Check sheet for the drawn part. Datum: minimum x, y, z corner. Units: mm. Coordinates: 2 decimals unless noted, no trailing zeros. Order: outer loops, then holes, each group sorted by start corner. A loop starts at its lowest first (then second) coordinate and runs counter-clockwise, first axis right, second up. Notation, with made-up numbers: M 15.25,61 L 37.25,61 A5 cw 37.25,67 Z; hole C -13,-22.75 d5. An arc over 180 degrees is marked long. Use one line per item in the form item = value. Start each with the question number.
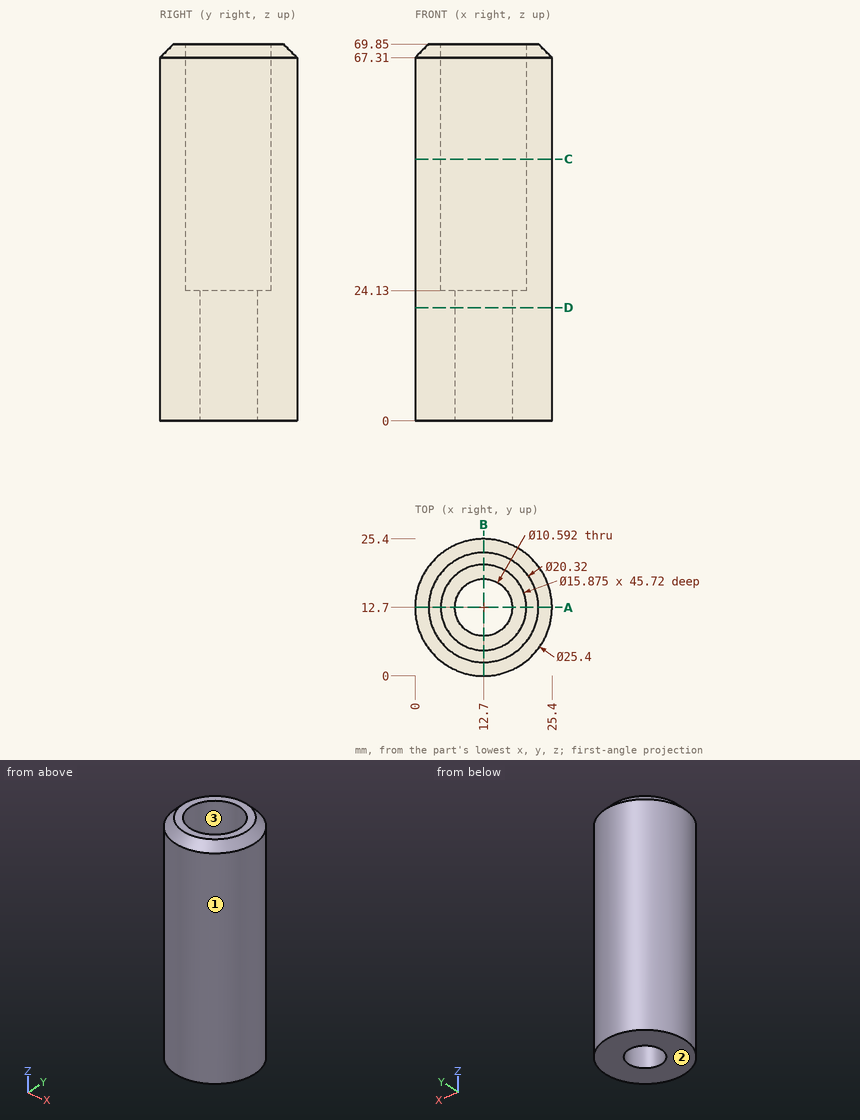
1. Cross-section at D-D on z = 21. Enter the section's corners in (x, y), and give its area (3 significant figures).
2. Depth check by flat-ended pin: P1, Ø12.5, axis at x = 12.7, y = 12.7, coming from the +Z side; P2, Ø5, axis at x = 20.5, z = 17.5, coming from the +Y side; P3, Ø5, axis at x = 17.5, z = 44, coming from the +Y side. Enter the tip coordinate at first touch or a pass-through.
3. Material ranges on line 1 along X through (y, z) = (12.5, 27.5) (1 decimal); line 2 along Y through (x, z) = (12.7, 45); line 3 along Y through (x, z) = (12.7, 15.5), recorded low to high.
4. Cross-section at C-C on z = 48.5. Enter the section's corners in (x, y) (1 decimal).
5. Release check for a two-part mould opening along X. For the marked faces 1, 2 and 3 record: pulls with the +X half, pulls with the -X half, needs draft (parallel to the pull), parting line crosses it, or undercut.
6. Cross-section at A-A on y = 12.7. Enter the section's corners in (x, z), and give its area (3 significant figures).
Final values:
q1.outline = C 12.7,12.7 d25.4; hole C 12.7,12.7 d10.59
q1.area = 419 mm2
q2.P1 = 24.13
q2.P2 = 24.24
q2.P3 = 25.19
q3.line_1 = 0 to 4.8, 20.6 to 25.4
q3.line_2 = 0 to 4.76, 20.64 to 25.4
q3.line_3 = 0 to 7.4, 18 to 25.4
q4.outline = C 12.7,12.7 d25.4; hole C 12.7,12.7 d15.9
q5.face_1 = parting line crosses it
q5.face_2 = needs draft
q5.face_3 = undercut
q6.outline = M 0,0 L 7.4,0 L 7.4,24.13 L 4.76,24.13 L 4.76,69.85 L 2.54,69.85 L 0,67.31 Z; M 18,0 L 25.4,0 L 25.4,67.31 L 22.86,69.85 L 20.64,69.85 L 20.64,24.13 L 18,24.13 Z
q6.area = 786 mm2
